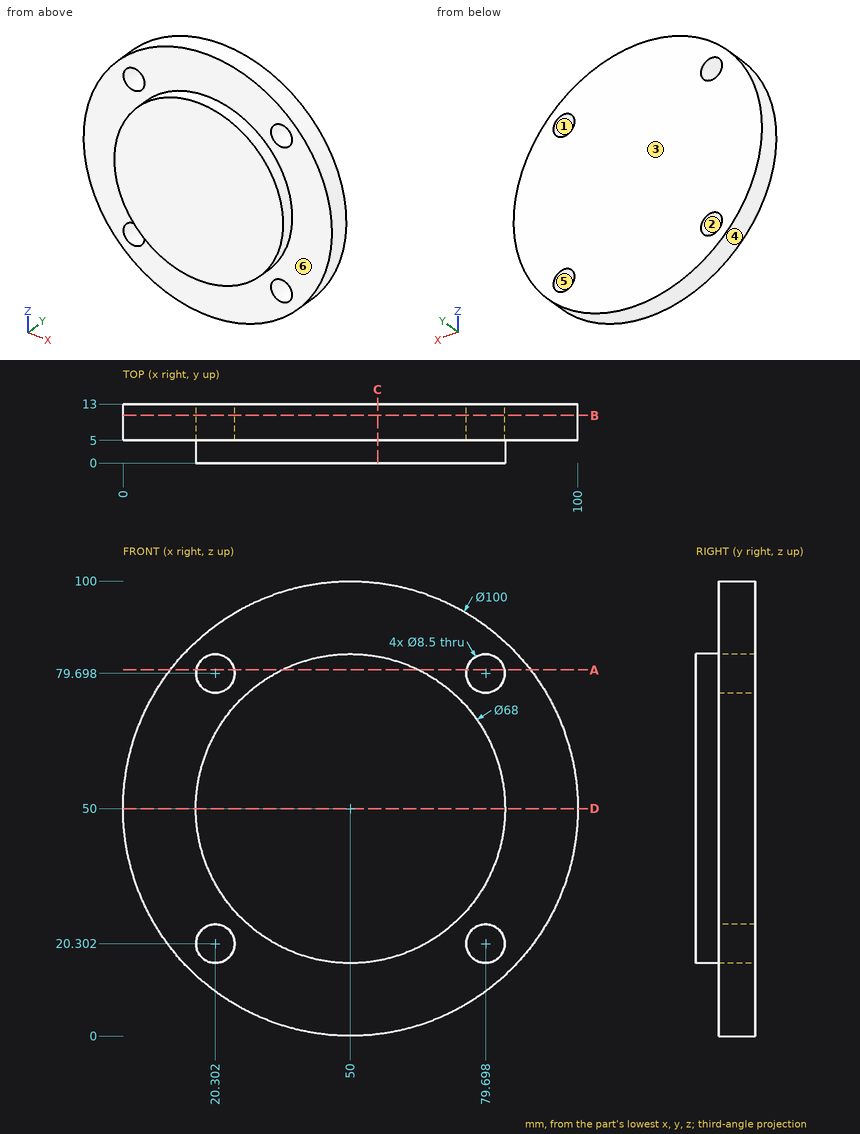
The figure shows three views and two pictorial views of one solid part (mm, origin at its lowest corner). Answer the questions. A direction names the side the tool comes from. Give positions to 0.01 mm unless a question says otherwise; leave off trailing zeros. Order: outer loops, then holes, each group sorted by start corner. A loop starts at its lowest first (then second) coordinate and runs counter-clockwise, first axis right, second up. Notation, with made-up numbers: (-34, 15) -> (-18, 15) arc R24 cw to (-18, 49) -> close; hole circle Ø5 at (-28, -29.75). An arc over 180 degrees is marked (long way). Answer as a JSON object with one key per item and string values. Group by question number.
Item 1: The part is cut by section B-B on y = 10.5. Write down the section's boundary in (x, z), and give its area (3 significant figures).
Item 2: The part is cut by section C-C on x = 56. Write down the section's boundary in (y, z).
Item 3: Flat-ended cylindrical pins translate along their axes: pin 1 (1 mm diameter, centred on x = 22.5, y = 2, fed in from +Z) (1 decimal); pin 2 (10 mm diameter, centred on x = 79.7, z = 20.3, fed in from -Y); pin 3 (1.5 mm diameter, centred on y = 6.5, z = 44, fed in from +X). Find the tip coordinate at first contact, or state that the pin passes through.
Item 4: Consider L1, parallel to Z at x = 78, y = 9.5 (1 decimal); L2, parallel to Y at x = 62, z = 95; L3, parallel to X at y = 3.5, z = 52. Determine where each line is inside the solid, lowest interval first. Write a range as from..to.
Item 5: Determine the mould class of the marked faces 1, 2, 3 and 4 for opening direction X: pulls with the +X half, pulls with the -X half, needs draft (parallel to the pull), parting line crosses it, or undercut.
Item 6: The part is cut by section A-A on z = 80.5. Write down the section's boundary in (x, y) (1 decimal).
Item 7: The part is cut by section D-D on z = 50. Write down the section's boundary in (x, y), and give its area (3 significant figures).
Item 8: A tool of negligible diameter and unlimited length cuts with its end or side. For the marked faces 5 and 6, from which of +Z, -Z, +X, -X, +Y, -Y can it reach the whole face along a straight path? Write none if from no direction.
Result set:
{
 "1": {"outline": "circle Ø100 at (50, 50); hole circle Ø8.5 at (20.3, 20.3); hole circle Ø8.5 at (20.3, 79.7); hole circle Ø8.5 at (79.7, 20.3); hole circle Ø8.5 at (79.7, 79.7)", "area": "7,630 mm²"},
 "2": {"outline": "(0, 16.53) -> (5, 16.53) -> (5, 0.36) -> (13, 0.36) -> (13, 99.64) -> (5, 99.64) -> (5, 83.47) -> (0, 83.47) -> close"},
 "3": {"pin 1": "z = 70.7", "pin 2": "y = 5", "pin 3": "x = 99.72"},
 "4": {"L1": "8.6..16.4, 24.2..75.8, 83.6..91.4", "L2": "5..13", "L3": "16.06..83.94"},
 "5": {"face 1": "undercut", "face 2": "undercut", "face 3": "needs draft", "face 4": "parting line crosses it"},
 "6": {"outline": "(10.4, 5) -> (16.1, 5) -> (16.1, 13) -> (10.4, 13) -> close; (24.5, 5) -> (35, 5) -> (35, 0) -> (65, 0) -> (65, 5) -> (75.5, 5) -> (75.5, 13) -> (24.5, 13) -> close; (83.9, 5) -> (89.6, 5) -> (89.6, 13) -> (83.9, 13) -> close"},
 "7": {"outline": "(0, 5) -> (16, 5) -> (16, 0) -> (84, 0) -> (84, 5) -> (100, 5) -> (100, 13) -> (0, 13) -> close", "area": "1,140 mm²"},
 "8": {"face 5": "+Y, -Y", "face 6": "-Y"}
}
